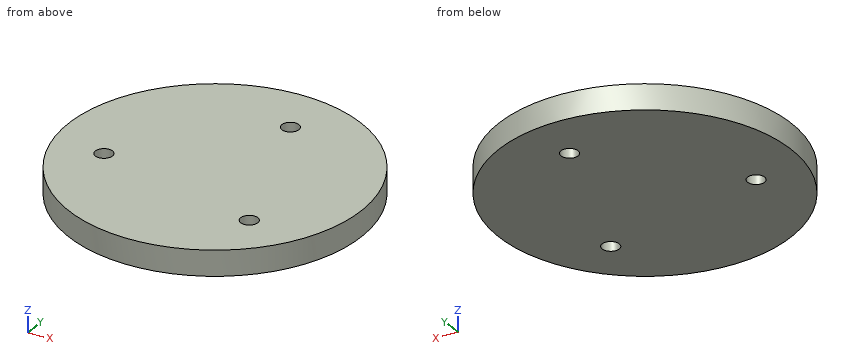
```python
from build123d import *

# Parameters (mm, degrees)
ESQUISSE1_R             = 57.5
BOSS_EXTRU_1_DEPTH      = 10
ECHELLE1_SCALE          = 2
ECHELLE2_SCALE          = 0.25
ESQUISSE2_R             = 1.6875
ENL_V_MAT_EXTRU_1_DEPTH = 10


with BuildPart() as part:
    # Esquisse1 → Boss.-Extru.1 (new body)
    with BuildSketch(Plane.XY):
        Circle(ESQUISSE1_R)
    extrude(amount=BOSS_EXTRU_1_DEPTH)


with BuildPart() as part_1:
    # Echelle1: scaled about (0, 0, 5)
    add(part.part.scale(ECHELLE1_SCALE).moved(Location((0, 0, -5))))


with BuildPart() as part_2:
    # Echelle2: scaled about (0, 0, 5)
    add(part_1.part.scale(ECHELLE2_SCALE).moved(Location((0, 0, 3.75))))

    # Esquisse2 → Enlèv. mat.-Extru.1 (cut)
    with BuildSketch(Plane(origin=(0, 0, 2.5), x_dir=(-1, 0, 0), z_dir=(0, 0, -1))):
        with Locations((-3.959214709, 18.22761283)):
            Circle(ESQUISSE2_R)
        with Locations((18.38283853, -5.330774337)):
            Circle(ESQUISSE2_R)
        with Locations((-14.213467184, -13.006989818)):
            Circle(ESQUISSE2_R)
    extrude(amount=-ENL_V_MAT_EXTRU_1_DEPTH, mode=Mode.SUBTRACT)


solid = part_2.part
```
Could you check a few things on this model? Use its own coordinates, in mm. Round coordinates to 2 decimals unless told otherwise and drop trailing zeros. Loops run counter-clockwise (first coordinate to the right, second up) from the corner with the lowest first, then second, coordinate; pieces in that order, holes last.
Q1. Please list where these lines run through material, in increasing order: L1, parallel to Y at x = 3, z = 6.65; L2, parallel to Y at x = -14, z = 6.3; L3, parallel to Y at x = -19, z = 6.7.
Q2. For P1, Ø2, axis at x = -18.38, y = -5.33, coming from the +Z side; P2, Ø3, axis at x = 7.5, z = 3.5, coming from the +Y side, each with a flat end and sliding along its axis, tell me the tip position at first contact or that it passes through.
Q3. I want a section at B-B (y = 7). Write out the boundary of the cut face in (x, z).
Q4. I want a section at A-A (x = -24.5). Write out the boundary of the cut face in (y, z), and give its area (3 significant figures).
Q5. I want a section at C-C (z = 5.8). Give the number of separate pieces and of enclosed holes in the cut face, and give its area (3 significant figures).
Answer below:
1. L1: y = -28.59 to 16.84, 19.62 to 28.59
1. L2: y = -25.11 to 25.11
1. L3: y = -21.58 to -6.9, -3.76 to 21.58
2. P1: passes through
2. P2: stops at y = 28.12
3. outline: (-27.88, 2.5) - (27.88, 2.5) - (27.88, 7.5) - (-27.88, 7.5) - close
4. outline: (-15.04, 2.5) - (15.04, 2.5) - (15.04, 7.5) - (-15.04, 7.5) - close
4. area: 150 mm2
5. separate pieces: 1
5. enclosed holes: 3
5. area: 2,570 mm2
